Verification items for the finished model (mm, model axes). A direction names the side the tool comes from. Coordinates: 2 decimals unless noted, no trailing zeros. Order: outer loops, then holes, each group sorted by start corner. A loop starts at its lowest first (then second) coordinate and runs counter-clockwise, first axis right, second up. Notation, with made-up numbers: (-15.75, -34) -> (18.25, -34) arc R14 ccw to (18.25, -30) -> close; hole circle Ø9 at (42.25, 6.25). An arc over 180 degrees is marked (long way). Write each question's results on one line, items separated by ' | '. Start each with the question number.
(1) Set-up check for faces 4 (the flat face through (0, 1, 0)), 5 (the flat face through (0, 0, -4)): record each of +Z, -Z, +X, -X, +Y, -Y from which the full face is reachable in a straight line by a thin tool's end or side.
(2) Thickness scan on probe 1 along Y at (x, z) = (4.5, 3.5); probe 2 along Z at (x, y) = (0, 1.2); probe 3 along Z at (x, y) = (0, 1.75). Record the ranges inside material, lowest first. Write a range as [from, to].
(3) Cross-section at C-C on z = -1.5. Enter the section's corners in (x, y), and give its area (3 significant figures).
(4) Draft check along Z on faces 1 (the cylindrical face through (-7.215, 1.699, -3.549)), 2 (the cylindrical face through (-5.994, 1.507, -0.264)), 3 (the cylindrical face through (-0.16, 0.49, -14.5)). Enter one of: +Z half, -Z half, draft (parallel to the pull), parting line (faces both ways), or undercut.
(5) Cross-section at B-B on y = 0.5. Enter the section's corners in (x, z), and give its area (3 significant figures).
(6) Cross-section at A-A on x = 0. Enter the section's corners in (y, z).
(7) Cross-section at D-D on y = 1.75. Enter the section's corners in (x, z).
(8) Go/stop test with a flat-tipped pin: pin 1 (3.5 mm diameter, centred on x = -1, z = -1.5, fed in from +Y). Record where the tip stops, or that it passes through.
```python
from build123d import *

# Parameters (mm, degrees)
BOSS_EXTRUDE2_DEPTH = 2
SKETCH3_R           = 6
CUT_EXTRUDE1_DEPTH  = 1
FILLET2_R           = 1


with BuildPart() as part:
    # Sketch2 → Boss-Extrude2 (new body)
    with BuildSketch(Plane(origin=(0, 0, 0), x_dir=(1, 0, 0), z_dir=(0, 1, 0))):
        with BuildLine():
            Line((-7.5, 0), (-7.5, 7))
            ThreePointArc((-7.5, 7), (0, 14.5), (7.5, 7))
            Line((7.5, 7), (7.5, 0))
            ThreePointArc((7.5, 0), (0, -7.5), (-7.5, 0))
        make_face()
    extrude(amount=BOSS_EXTRUDE2_DEPTH)

    # Sketch3 → Cut-Extrude1 (cut)
    with BuildSketch(Plane(origin=(0, 2, 0), x_dir=(1, 0, 0), z_dir=(0, 1, 0))):
        Circle(SKETCH3_R)
    extrude(amount=-CUT_EXTRUDE1_DEPTH, mode=Mode.SUBTRACT)

    # Fillet2
    fillet2_edges = [part.edges().sort_by_distance(p)[0] for p in [
        (0, 2, -14.5),
        (-7.5, 2, -3.5),
        (0, 2, 7.5),
        (7.5, 2, -3.5),
    ]]
    fillet(fillet2_edges, radius=FILLET2_R)


solid = part.part
```
Results are:
1) face 4: +Y | face 5: +Z, -Z, +X, -X, -Y
2) probe 1: y = [0, 1] | probe 2: z = [-14.48, -6], [6, 7.48] | probe 3: z = [-14.16, -6], [6, 7.16]
3) outline: (-7.5, 0) -> (7.5, 0) -> (7.5, 1) arc R1 ccw to (6.5, 2) -> (5.81, 2) -> (5.81, 1) -> (-5.81, 1) -> (-5.81, 2) -> (-6.5, 2) arc R1 ccw to (-7.5, 1) -> close | area: 18.0 mm2
4) face 1: draft | face 2: undercut | face 3: -Z half
5) outline: (-7.5, -7) arc R7.5 ccw to (7.5, -7) -> (7.5, 0) arc R7.5 ccw to (-7.5, 0) -> close | area: 282 mm2
6) outline: (0, -14.5) -> (1, -14.5) arc R1 ccw to (2, -13.5) -> (2, -6) -> (1, -6) -> (1, 6) -> (2, 6) -> (2, 6.5) arc R1 ccw to (1, 7.5) -> (0, 7.5) -> close
7) outline: (-7.16, -7) arc R7.16 ccw to (7.16, -7) -> (7.16, 0) arc R7.16 ccw to (-7.16, 0) -> close; hole circle Ø12 at (0, 0)
8) pin 1: stops at y = 1
